The figure shows three views and two pictorial views of one solid part (mm, origin at its lowest corner). Answer the questions. A direction names the side the tool comes from. Give positions to 0.01 mm unless a question says otherwise; leave off trailing zeros. Order: outer loops, then holes, each group sorted by start corner. A loop starts at its lowest first (then second) coordinate and runs counter-clockwise, first axis right, second up. Notation, with made-up numbers: (24.25, 44.25) - (67.25, 44.25) arc R16 ccw to (67.25, 62.25) - close; hole circle Ø4 at (56.25, -28.75). An arc over 180 degrees is marked (long way). Answer as a JSON object with one key per item and string values. Group by question number.
Q1. Given pin 1 (1 mm diameter, centred on x = 19.5, z = 5.5, fed in from -Y), flat-ended and moving along its own axis, determine where the tip first touches the part or whether it passes through.
Q2. The mould has two halves that part along Y. Classify the marked faces 1, 2, 3 and 4: released by +Y, released by -Y, zero draft, split by the parting line, or undercut.
Q3. A cutting plane is placed at B-B, the plane x = 19. Give the vertices of the cut face in (y, z).
Q4. A cutting plane is placed at A-A, the plane z = 5.5. Give the vertices of the cut face in (x, y), and give its area (3 significant figures).
Q5. For the marked faces 5 and 6, determine the directions among +Z, -Z, +X, -X, +Y, -Y from which every point of the face is accessible in a straight line to the end or side of a thin tool.
Q6. A cutting plane is placed at C-C, the plane z = 7.5. Count the separate pieces of the cut face and the enclosed holes in it, and give its area (3 significant figures).
Q7. A cutting plane is placed at D-D, the plane x = 11. Give the vertices of the cut face in (y, z), and give its area (3 significant figures).
Q8. Consider line 1 (X direction, y = 0.35, z = 7.5); line 2 (Z direction, x = 30, y = 6.25). Determine where each line is inside the solid, lowest interval first.
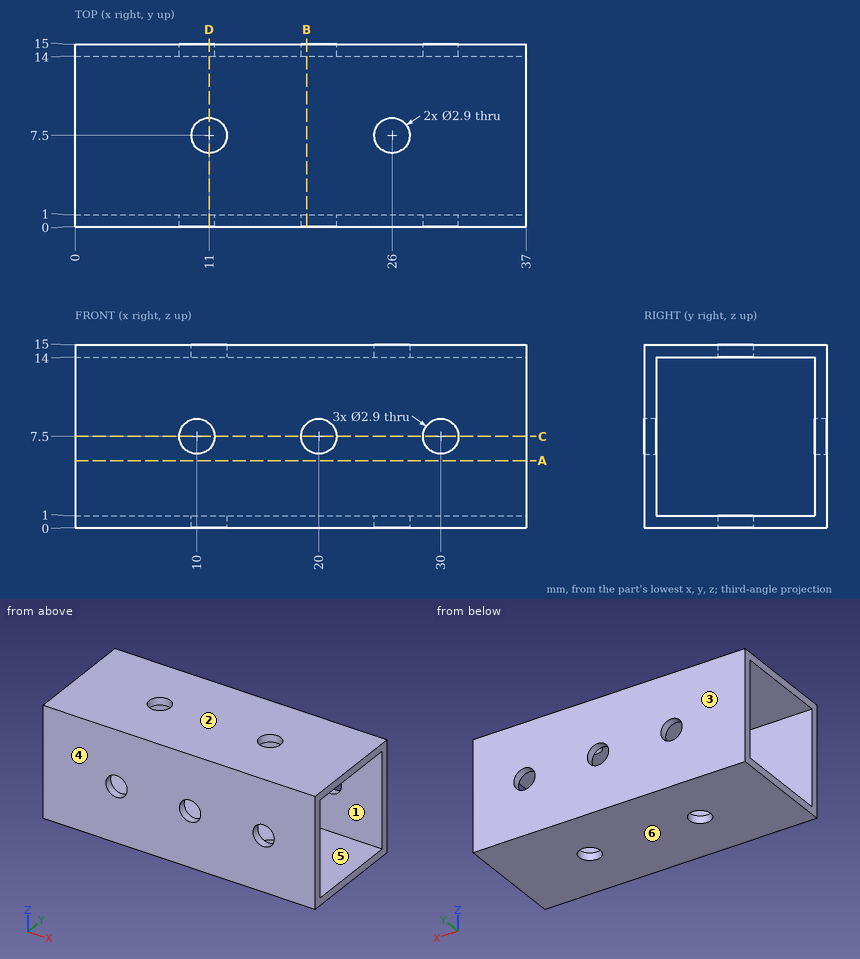
Reply:
{
 "1": {"pin 1": "stops at y = 0"},
 "2": {"face 1": "undercut", "face 2": "zero draft", "face 3": "released by +Y", "face 4": "released by -Y"},
 "3": {"outline": "(0, 0) - (15, 0) - (15, 6.45) - (14, 6.45) - (14, 1) - (1, 1) - (1, 6.45) - (0, 6.45) - close; (0, 8.55) - (1, 8.55) - (1, 14) - (14, 14) - (14, 8.55) - (15, 8.55) - (15, 15) - (0, 15) - close"},
 "4": {"outline": "(0, 0) - (37, 0) - (37, 1) - (0, 1) - close; (0, 14) - (37, 14) - (37, 15) - (0, 15) - close", "area": "74.0 mm^2"},
 "5": {"face 5": "+X, -X", "face 6": "-Z, +X, -X, +Y, -Y"},
 "6": {"separate pieces": "8", "enclosed holes": "0", "area": "56.6 mm^2"},
 "7": {"outline": "(0, 0) - (6.05, 0) - (6.05, 1) - (1, 1) - (1, 6.45) - (0, 6.45) - close; (0, 8.55) - (1, 8.55) - (1, 14) - (6.05, 14) - (6.05, 15) - (0, 15) - close; (8.95, 0) - (15, 0) - (15, 6.45) - (14, 6.45) - (14, 1) - (8.95, 1) - close; (8.95, 14) - (14, 14) - (14, 8.55) - (15, 8.55) - (15, 15) - (8.95, 15) - close", "area": "46.0 mm^2"},
 "8": {"line 1": "x = 0 to 8.55, 11.45 to 18.55, 21.45 to 28.55, 31.45 to 37", "line 2": "z = 0 to 1, 14 to 15"}
}
